```python
from build123d import *

# Parameters (mm, degrees)
CROQUIS1_R                 = 4.9
CROQUIS1_R_2               = 2.9
SALIENTE_EXTRUIR1_DEPTH    = 4.6
CORTAR_EXTRUIR2_DEPTH      = 0.75
CORTAR_EXTRUIR2_DEPTH_BACK = 0.75
CROQUIS2_W                 = 2.8
CROQUIS2_H                 = 4.6
CROQUIS4_R                 = 1.65
SALIENTE_EXTRUIR2_DEPTH    = 2
SALIENTE_EXTRUIR3_DEPTH    = 8
CORTAR_EXTRUIR3_DEPTH      = 19.912045786
CORTAR_EXTRUIR3_DEPTH_BACK = 19.912045786
CROQUIS6_R                 = 1.65
CHAFL_N1_SIZE              = 0.5


with BuildPart() as part:
    # Croquis1 → Saliente-Extruir1 (new body)
    with BuildSketch(Plane.XY):
        Circle(CROQUIS1_R)
        Circle(CROQUIS1_R_2, mode=Mode.SUBTRACT)
    extrude(amount=SALIENTE_EXTRUIR1_DEPTH)

    # Croquis2 → Cortar-Extruir2 (cut, two sides: drawn at the far end of the back side and taken through both)
    with BuildSketch(Plane(origin=(0, 0, 0), x_dir=(1, 0, 0), z_dir=(0, 1, 0)).offset(-CORTAR_EXTRUIR2_DEPTH_BACK)):
        with Locations((3.6, -2.3)):
            Rectangle(CROQUIS2_W, CROQUIS2_H)
    extrude(amount=CORTAR_EXTRUIR2_DEPTH + CORTAR_EXTRUIR2_DEPTH_BACK, mode=Mode.SUBTRACT)



with BuildPart() as body_2:
    # Croquis4 → Saliente-Extruir2 (new body)
    with BuildSketch(Plane(origin=(0, -0.75, 0), x_dir=(1, 0, 0), z_dir=(0, 1, 0))):
        Polygon((4.842261868, -4.6), (10.142261868, -4.6), (10.142261868, 0), (4.842261868, 0), (2.801338966, 0), (2.801338966, -4.6), align=None)
        with Locations(Location((7.492261868, -2.3, 0), (0, 0, 270))):
            Circle(CROQUIS4_R, mode=Mode.SUBTRACT)
    extrude(amount=-SALIENTE_EXTRUIR2_DEPTH)


with BuildPart() as body_3:
    # Simetría3: mirrored copy
    add(body_2.part.mirror(Plane.ZX))


with BuildPart() as part_1:
    add(part.part)

    add(body_2.part)  # Saliente-Extruir3 merges body 2

    add(body_3.part)  # Saliente-Extruir3 merges body 3
    # Croquis5 → Saliente-Extruir3 (add)
    with BuildSketch(Plane.XY.offset(4.6)):
        with BuildLine():
            ThreePointArc((2.801338966, -0.75), (-2.9, 0), (2.801338966, 0.75))
            Line((2.801338966, 0.75), (4.842261868, 0.75))
            ThreePointArc((4.842261868, 0.75), (-4.9, 0), (4.842261868, -0.75))
            Line((4.842261868, -0.75), (2.801338966, -0.75))
        make_face()
        with BuildLine():
            Line((-2.829016319, 4.9), (-4.243524531, 2.449999908))
            ThreePointArc((-4.243524531, 2.449999908), (-2.450000051, 4.243524449), (-1.2e-08, 4.9))
            Line((-1.2e-08, 4.9), (-2.829016319, 4.9))
        make_face()
        with BuildLine():
            Line((-5.658032638, 0), (-4.243524553, -2.449999871))
            ThreePointArc((-4.243524553, -2.449999871), (-4.9, 2.1e-08), (-4.243524531, 2.449999908))
            Line((-4.243524531, 2.449999908), (-5.658032638, 0))
        make_face()
        with BuildLine():
            Line((-2.829016319, -4.9), (-1.5e-08, -4.9))
            ThreePointArc((-1.5e-08, -4.9), (-2.450000071, -4.243524438), (-4.243524553, -2.449999871))
            Line((-4.243524553, -2.449999871), (-2.829016319, -4.9))
        make_face()
        with BuildLine():
            Line((-1.5e-08, -4.9), (2.829016319, -4.9))
            Line((2.829016319, -4.9), (4.24352445, -2.45000005))
            ThreePointArc((4.24352445, -2.45000005), (2.449999969, -4.243524497), (-1.5e-08, -4.9))
        make_face()
        with BuildLine():
            Line((2.829016319, 4.9), (-1.2e-08, 4.9))
            ThreePointArc((-1.2e-08, 4.9), (2.450000039, 4.243524456), (4.243524529, 2.449999913))
            Line((4.243524529, 2.449999913), (2.829016319, 4.9))
        make_face()
        with BuildLine():
            Line((4.842261868, 0.75), (5.225019936, 0.75))
            Line((5.225019936, 0.75), (4.243524529, 2.449999913))
            ThreePointArc((4.243524529, 2.449999913), (4.621728956, 1.627765788), (4.842261868, 0.75))
        make_face()
        with BuildLine():
            ThreePointArc((4.842261868, -0.75), (4.621728929, -1.627765863), (4.24352445, -2.45000005))
            Line((4.24352445, -2.45000005), (5.225019936, -0.75))
            Line((5.225019936, -0.75), (4.842261868, -0.75))
        make_face()
    extrude(amount=SALIENTE_EXTRUIR3_DEPTH)

    # Croquis6 → Cortar-Extruir3 (cut, two sides: drawn at the far end of the back side and taken through both)
    with BuildSketch(Plane.XZ.offset(4.9).offset(-CORTAR_EXTRUIR3_DEPTH_BACK)):
        with Locations((0, 8.6)):
            Circle(CROQUIS6_R)
    extrude(amount=CORTAR_EXTRUIR3_DEPTH + CORTAR_EXTRUIR3_DEPTH_BACK, mode=Mode.SUBTRACT)

    # Chaflán1
    # the kernel refuses this chamfer: 0.5 mm, written as the material it adds along each edge
    with BuildSketch(Plane(origin=(0, 0, 4.6), x_dir=(0, 1, 0), z_dir=(1, 0, 0))) as chafl_n1_piece_1_section:
        Polygon((4.9 + CHAFL_N1_SIZE, 0), (4.9, -CHAFL_N1_SIZE), (4.9, 0), align=None)
    chafl_n1_piece_1 = revolve(axis=Axis((0, 0, 4.6), (0, 0, 1)), revolution_arc=59.999998828, mode=Mode.PRIVATE)
    chafl_n1_piece_1 = split(chafl_n1_piece_1, bisect_by=Plane(origin=(-2.470137352, 4.9, 4.415231156), z_dir=(0, -1, 0)), keep=Keep.TOP, mode=Mode.PRIVATE)
    chafl_n1_piece_1 = split(chafl_n1_piece_1, bisect_by=Plane(origin=(-3.008455802, 4.589201698, 4.415231156), z_dir=(0.8660254037844386, -0.5000000000000002, 0)), keep=Keep.TOP, mode=Mode.PRIVATE)
    add(chafl_n1_piece_1)
    with BuildSketch(Plane(origin=(0, 0, 4.6), x_dir=(-0.8660253935532619, 0.5000000177209175, 0), z_dir=(0.5000000177209175, 0.8660253935532619, 0))) as chafl_n1_piece_2_section:
        Polygon((4.9 + CHAFL_N1_SIZE, 0), (4.9, -CHAFL_N1_SIZE), (4.9, 0), align=None)
    chafl_n1_piece_2 = revolve(axis=Axis((0, 0, 4.6), (0, 0, 1)), revolution_arc=59.99999929, mode=Mode.PRIVATE)
    chafl_n1_piece_2 = split(chafl_n1_piece_2, bisect_by=Plane(origin=(-5.478593155, 0.310798302, 4.415231156), z_dir=(0.8660254037844386, -0.5000000000000002, 0)), keep=Keep.TOP, mode=Mode.PRIVATE)
    chafl_n1_piece_2 = split(chafl_n1_piece_2, bisect_by=Plane(origin=(-5.478593155, -0.310798302, 4.415231156), z_dir=(0.8660254037844386, 0.5000000000000002, 0)), keep=Keep.TOP, mode=Mode.PRIVATE)
    add(chafl_n1_piece_2)
    with BuildSketch(Plane(origin=(0, 0, 4.6), x_dir=(-0.8660254202095417, -0.4999999715508861, 0), z_dir=(-0.4999999715508861, 0.8660254202095417, 0))) as chafl_n1_piece_3_section:
        Polygon((4.9 + CHAFL_N1_SIZE, 0), (4.9, -CHAFL_N1_SIZE), (4.9, 0), align=None)
    chafl_n1_piece_3 = revolve(axis=Axis((0, 0, 4.6), (0, 0, 1)), revolution_arc=60.000001882, mode=Mode.PRIVATE)
    chafl_n1_piece_3 = split(chafl_n1_piece_3, bisect_by=Plane(origin=(-3.008455802, -4.589201698, 4.415231156), z_dir=(0.8660254037844386, 0.5000000000000002, 0)), keep=Keep.TOP, mode=Mode.PRIVATE)
    chafl_n1_piece_3 = split(chafl_n1_piece_3, bisect_by=Plane(origin=(-2.470137352, -4.9, 4.415231156), z_dir=(0, 1, 0)), keep=Keep.TOP, mode=Mode.PRIVATE)
    add(chafl_n1_piece_3)
    with BuildSketch(Plane(origin=(0, 0, 4.6), x_dir=(0, -1, 0), z_dir=(-1, 0, 0))) as chafl_n1_piece_4_section:
        Polygon((4.9 + CHAFL_N1_SIZE, 0), (4.9, -CHAFL_N1_SIZE), (4.9, 0), align=None)
    chafl_n1_piece_4 = revolve(axis=Axis((0, 0, 4.6), (0, 0, 1)), revolution_arc=70.897169979, mode=Mode.PRIVATE)
    chafl_n1_piece_4 = split(chafl_n1_piece_4, bisect_by=Plane(origin=(2.466837368, -4.9, 4.415358811), z_dir=(0, 1, 0)), keep=Keep.TOP, mode=Mode.PRIVATE)
    add(chafl_n1_piece_4)
    with BuildSketch(Plane(origin=(0, 0, 4.6), x_dir=(0.9449327486717788, 0.3272645726130418, 0), z_dir=(0.3272645726130418, -0.9449327486717788, 0))) as chafl_n1_piece_5_section:
        Polygon((4.9 + CHAFL_N1_SIZE, 0), (4.9, -CHAFL_N1_SIZE), (4.9, 0), align=None)
    chafl_n1_piece_5 = revolve(axis=Axis((0, 0, 4.6), (0, 0, 1)), revolution_arc=70.897169979, mode=Mode.PRIVATE)
    chafl_n1_piece_5 = split(chafl_n1_piece_5, bisect_by=Plane(origin=(3.940959453, 4.9, 4.468069459), z_dir=(0, -1, 0)), keep=Keep.TOP, mode=Mode.PRIVATE)
    add(chafl_n1_piece_5)


solid = part_1.part
```
Can you work these out from the model? Positions are in its coordinate system, mm. A direction names the side the tool comes from. Round coordinates to 2 decimals unless told otherwise and drop trailing zeros. Loops run counter-clockwise (first coordinate to the right, second up) from the corner with the lowest first, then second, coordinate; pieces in that order, holes last. Notation, with made-up numbers: M -20.75,-22.75 L 37.25,-22.75 A24 ccw 37.25,5.25 Z; hole C 66,79 d9. An arc over 180 degrees is marked long. Answer in a Markdown table with one row per item.
1. Thinking about a two-plate mould opening in X: for faces 1 (the face through (1, 4.9, 7)), 2 (the face through (1.524, 3.66, 7.968)), 3 (the face through (10.142, 2, 2)), which applies, pulls with the +X half, pulls with the -X half, needs draft (parallel to the pull), parting line crosses it, or undercut?
Established:
| item | result |
|---|---|
| face 1 | needs draft |
| face 2 | undercut |
| face 3 | pulls with the +X half |
2. If we section it at B-B, the plane x = 8.75: Please give me the cut outline in (y, z), plus the area to 3 significant figures.
Established:
| item | result |
|---|---|
| outline | M -2.75,0 L -0.75,0 L -0.75,1.23 L -2.75,1.23 Z; M -2.75,3.37 L -0.75,3.37 L -0.75,4.6 L -2.75,4.6 Z; M 0.75,0 L 2.75,0 L 2.75,1.23 L 0.75,1.23 Z; M 0.75,3.37 L 2.75,3.37 L 2.75,4.6 L 0.75,4.6 Z |
| area | 9.86 mm² |
3. If we section it at D-D, the plane y = 2: Give the number of separate pieces and of enclosed holes in the cut face, plus the area to 3 significant figures.
Established:
| item | result |
|---|---|
| separate pieces | 2 |
| enclosed holes | 1 |
| area | 77.8 mm² |
4. On a 3-axis mill with a long thin cutter (end or side, diameter ignored), from which of +Z, -Z, +X, -X, +Y, -Y can I reach the whole of each face in a straight line? I mean faces 4 (the face through (5, 0.75, 5)), 5 (the face through (5.7, 2.75, 2.8)), 6 (the face through (-4.897, 0.175, 2.021)), 7 (the face through (5.7, -2.75, 2.8)), 8 (the face through (7, 2, 4.6)). Say none if no direction works.
Established:
| item | result |
|---|---|
| face 4 | +Z, -Z, +X |
| face 5 | -Z, +X, +Y |
| face 6 | -Z |
| face 7 | -Z, +X, -Y |
| face 8 | +Z, +X, +Y |
5. If we section it at A-A, the plane z = 8.6: Please give me the cut outline in (x, y).
Established:
| item | result |
|---|---|
| outline | M -5.66,0 L -2.83,-4.9 L -1.65,-4.9 L -1.65,-2.38 A2.9 cw -1.65,2.38 L -1.65,4.9 L -2.83,4.9 Z; M 1.65,-4.9 L 2.83,-4.9 L 5.23,-0.75 L 2.8,-0.75 A2.9 cw 1.65,-2.38 Z; M 1.65,2.38 A2.9 cw 2.8,0.75 L 5.23,0.75 L 2.83,4.9 L 1.65,4.9 Z |
6. If we section it at C-C, the plane z = 5: Please give me the cut outline in (x, y).
Established:
| item | result |
|---|---|
| outline | M -5.66,0 L -2.83,-4.9 L 2.83,-4.9 L 5.23,-0.75 L 2.8,-0.75 A2.9 cw long 2.8,0.75 L 5.23,0.75 L 2.83,4.9 L -2.83,4.9 Z |
7. Please list where these lines run through material, in increasing order: line 1 (X direction, y = -1.6, z = 2.3); line 2 (Z direction, x = 0, y = 3.7); line 3 (Y direction, x = 4.25, z = 2.5). Write a range as from..to.
Established:
| item | result |
|---|---|
| line 1 | -4.63..-2.42, 2.42..5.84, 9.14..10.14 |
| line 2 | 0..6.95, 10.25..12.6 |
| line 3 | -2.75..-0.75, 0.75..2.75 |
8. I'm going to push flat-ended pins straight in: pin 1 Ø1.1 at (x, y) = (6, 2) entering from +Z; pin 2 Ø0.5 at (x, y) = (2.5, -5) entering from -Z; pin 3 Ø3 at (x, z) = (2, 2.5) entering from +Y. Where does each tip first touch, or does it pass through?
Established:
| item | result |
|---|---|
| pin 1 | z = 4.6 |
| pin 2 | z = 4.54 |
| pin 3 | y = 4.87 |
